Model file for the job. Use its own axes, mm. Give positions to 0.01 mm unless a question says otherwise; leave off trailing zeros. Loops run counter-clockwise (first coordinate to the right, second up) from the corner with the lowest first, then second, coordinate; pieces in that order, holes last. Notation, with made-up numbers: (36.5, 23.5) -> (50.5, 23.5) arc R11 cw to (50.5, 44.5) -> close; hole circle Ø4 at (-26, 16.25). An arc over 180 degrees is marked (long way). Use CSV: the item, a comma, the result in double quotes. Start each with the question number.
(1) Cut at B-B on y = 109.5. Write the cut outline in (x, z).
(2) Cut at A-A on z = 4.25. Write the cut outline in (x, y) (3 decimals), then the cut area to 3 significant figures.
(3) Pull direction Y, two halves, no side cores. Call faces 1 (the cylindrical face through (-74.11, 125.57, 0.09)), 2 (the flat face through (-79.332, -173.372, -0.091)), 3 (the flat face through (-2, 4, 6.5)): pulls with the +Y half, pulls with the -Y half, needs draft (parallel to the pull), parting line crosses it, or undercut.
(4) Drill centre lines: probe 1 along Y at (x, z) = (-56.5, 2.5); probe 2 along Y at (x, z) = (-66.5, 2.25); probe 3 along Y at (x, z) = (-69, -1). Where is each one in solid material? Low to high.
(5) Cut at C-C on x = -46.5. Write the cut outline in (y, z).
(6) Flat gauge pins, fed straight in: pin 1 (20.5 mm diameter, centred on x = -71.723, y = 203.108, fed in from +Z); pin 2 (1 mm diameter, centred on y = -179.5, z = -4.5, fed in from -X); pin 3 (6 mm diameter, centred on y = -69.5, z = -4, fed in from +X); pin 4 (16 mm diameter, centred on x = -71.723, y = 69.504, fed in from -Z). Where does each tip first touch, or does it go through?
Autodesk Inventor part; units mm, degrees
ref_plane "YZ Plane" through (0, 0, 0) normal (1, 0, 0) x (0, 1, 0)
ref_plane "XZ Plane" through (0, 0, 0) normal (0, 1, 0) x (-1, 0, 0)
ref_plane "XY Plane" through (0, 0, 0) normal (0, 0, 1) x (1, 0, 0)
sketch "Sketch1" plane through (0, 0, 0) normal (0, 0, 1) x (1, 0, 0)
  line L0 (-127.68, 259.036) -> (-127.68, -85.275)
  line L1 (-127.68, 259.036) -> (47.477, 259.036)
  line L2 (127.68, -259.036) -> (-32.32, -259.036)
  line L3 (-32.32, -259.036) -> (-127.68, -85.275)
  line L4 (127.68, -259.036) -> (127.68, -145.836)
  line L5 (127.68, -145.836) -> (47.477, 259.036)
  point P0 (0, 0)
  dimension "d6" = 344.311
  dimension "d7" = 175.157
  dimension "d9" = 160
  dimension "d10" = 113.2
extrude "Extrusion1" add sketch "Sketch1" along normal mid plane 13
sketch "Sketch2" plane through (0, 0, 6.5) normal (0, 0, 1) x (1, 0, 0)
  circle A0 centre (-71.723, 203.108) radius 9
  circle A1 centre (-71.723, 69.504) radius 9
  circle A2 centre (-71.723, 136.306) radius 11
  line L0 (-87.483, 152.066) -> (-55.963, 152.066)
  line L1 (-55.963, 152.066) -> (-55.963, 120.546)
  line L2 (-55.963, 120.546) -> (-87.483, 120.546)
  line L3 (-87.483, 120.546) -> (-87.483, 152.066)
  line L4 (-87.483, 152.066) -> (-55.963, 120.546) construction
  line L5 (-55.963, 152.066) -> (-87.483, 120.546) construction
  circle A3 centre (-87.483, 152.066) radius 2.95
  circle A4 centre (-55.963, 152.066) radius 2.95
  circle A5 centre (-55.963, 120.546) radius 2.95
  circle A6 centre (-87.483, 120.546) radius 2.95
  line L6 (47.477, 259.036) -> (-127.68, 259.036)
  line L7 (-127.68, 259.036) -> (-127.68, -85.275)
  point P0 (0, 0)
  point P1 (-71.723, 136.306)
  dimension "d25" = 22
  dimension "d26" = 66.802
  dimension "d31" = 31.52
  dimension "d32" = 31.52
  dimension "d35" = 5.9
  dimension "d39" = 66.802
  dimension "d40" = 55.928
  dimension "d41" = 55.957
  dimension "d42" = 5.9
extrude "Extrusion3" cut sketch "Sketch2" against normal blind 25.4 contours A0 | A1 | A2 | L3 A3 L0 | L0 A3 L3 | A4 L1 L0 | L0 L1 A4 | A6 L2 L3 | L3 L2 A6 | A5 L2 L1 | L1 L2 A5
equation "\"d32\" = d31"
properties part number "CNC-Y-axis- side plates with stepper"
Check result:
1,outline,"(-127.68, -6.5) -> (77.1, -6.5) -> (77.1, 6.5) -> (-127.68, 6.5) -> close"
2,outline,"(-127.68, -85.275) -> (-32.32, -259.036) -> (127.68, -259.036) -> (127.68, -145.836) -> (47.477, 259.036) -> (-127.68, 259.036) -> close; hole circle Ø5.9 at (-87.483, 120.546); hole circle Ø5.9 at (-87.483, 152.066); hole circle Ø22 at (-71.723, 136.306); hole circle Ø18 at (-71.723, 69.504); hole circle Ø18 at (-71.723, 203.108); hole circle Ø5.9 at (-55.963, 120.546); hole circle Ø5.9 at (-55.963, 152.066)"
2,area,"107,000 mm²"
3,face 1,"undercut"
3,face 2,"pulls with the -Y half"
3,face 3,"needs draft"
4,probe 1,"-214.98 to 117.65, 123.45 to 149.17, 154.97 to 259.04"
4,probe 2,"-196.75 to 62.17, 76.83 to 126.63, 145.99 to 195.78, 210.44 to 259.04"
4,probe 3,"-192.2 to 60.93, 78.08 to 125.65, 146.96 to 194.53, 211.69 to 259.04"
5,outline,"(-233.2, -6.5) -> (259.04, -6.5) -> (259.04, 6.5) -> (-233.2, 6.5) -> close"
6,pin 1,"z = 6.5"
6,pin 2,"x = -76.24"
6,pin 3,"x = 113.15"
6,pin 4,"through"
